Solid Edge part; units mm, degrees
sketch "Sketch1" plane through (0, 0, 0) normal (0, -1, 0) x (1, 0, 0)
  line L0 (-47.0022, 489.0599) -> (-22.0022, 514.0599)
  line L1 (-22.0022, 514.0599) -> (-22.0022, 81.0447)
  line L2 (-22.0022, 81.0447) -> (162.9162, 149.0358)
  line L3 (197.0498, 56.2011) -> (162.9162, 149.0358)
  line L4 (-113.6611, -58.0415) -> (197.0498, 56.2011)
  line L5 (-113.6611, -58.0415) -> (-140.1715, 14.0599)
  line L6 (-522.0022, 14.0599) -> (-140.1715, 14.0599)
  line L7 (-497.0022, 39.0599) -> (-522.0022, 14.0599)
  line L8 (-497.0022, 39.0599) -> (-147.0022, 39.0599)
  line L9 (-47.0022, 139.0599) -> (-147.0022, 39.0599)
  line L10 (-47.0022, 139.0599) -> (-47.0022, 489.0599)
  dimension "D1" = 497.0022
extrude "Protrusion1" add sketch "Sketch1" along normal blind 10
sketch "Sketch2" plane through (-272.0022, -10, 264.0599) normal (0, -1, 0) x (0, 0, 1)
  line L0 (-265.7843, 265.7843) -> (-209.2157, 209.2157)
  line L1 (-209.2157, 209.2157) -> (-202.1447, 216.2868)
  line L2 (-202.1447, 216.2868) -> (-258.7132, 272.8553)
  line L3 (-258.7132, 272.8553) -> (-265.7843, 265.7843)
  line L4 (209.2157, -209.2157) -> (265.7843, -265.7843)
  line L5 (265.7843, -265.7843) -> (272.8553, -258.7132)
  line L6 (272.8553, -258.7132) -> (216.2868, -202.1447)
  line L7 (216.2868, -202.1447) -> (209.2157, -209.2157)
  dimension "D1" = 265.7843
  dimension "D2" = 272.8553
  dimension "D3" = 209.2157
  dimension "D4" = 202.1447
extrude "ExtrudedProtrusion_2" add sketch "Sketch2" against normal blind 80
sketch "Sketch3" plane through (-173.9038, -10, 239.4369) normal (0, -1, 0) x (1, 0, 0)
  line L0 (289.8917, -107.6558) -> (324.0253, -200.4904)
  line L1 (324.0253, -200.4904) -> (370.9537, -183.2357)
  line L2 (370.9537, -183.2357) -> (336.8201, -90.401)
  line L3 (336.8201, -90.401) -> (289.8917, -107.6558)
  dimension "D1" = 336.8201
  dimension "D2" = 370.9537
extrude "ExtrudedProtrusion_3" add sketch "Sketch3" along normal blind 50
sketch "Sketch4" plane through (-66.322, 10, 476.8112) normal (-0.7071068, 0, -0.7071068) x (0, -1, 0)
  line L0 (20, 5) -> (39.0788, 11)
  line L1 (39.0788, 11) -> (39.0788, 1)
  line L2 (39.0788, 1) -> (20, -5)
  line L3 (20, -5) -> (20, 5)
  line L4 (-60, 5) -> (-79.0788, 11)
  line L5 (-79.0788, 11) -> (-79.0788, 1)
  line L6 (-79.0788, 1) -> (-60, -5)
  line L7 (-60, 5) -> (-60, -5)
  dimension "D1" = 79.0788
  dimension "D2" = 79.0788
  dimension "D3" = 79.0788
extrude "ExtrudedProtrusion_4" add sketch "Sketch4" against normal blind 80
sketch "Sketch5" plane through (-541.322, 30, 1.8112) normal (-0.7071068, 0, -0.7071068) x (0, -1, 0)
  line L0 (-40, 5) -> (-59.0788, 11)
  line L1 (-59.0788, 11) -> (-59.0788, 1)
  line L2 (-59.0788, 1) -> (-40, -5)
  line L3 (-40, -5) -> (-40, 5)
  line L4 (40, 5) -> (40, -5)
  line L5 (40, -5) -> (59.0788, 1)
  line L6 (59.0788, 1) -> (59.0788, 11)
  line L7 (59.0788, 11) -> (40, 5)
extrude "ExtrudedProtrusion_5" add sketch "Sketch5" against normal blind 80
sketch "Sketch6" plane through (133.0546, -35, 85.3638) normal (-0.9385681, 0, -0.3450941) x (0, -1, 0)
  line L0 (25, 49.4555) -> (25, -49.4555)
  line L1 (25, -49.4555) -> (7.5593, -49.4555)
  line L2 (7.5593, -49.4555) -> (25, 49.4555)
extrude "Cutout1" cut sketch "Sketch6" against normal through all
The listing builds one solid part. Answer for the finished solid, in the listing's coordinates (mm). A direction names the side the tool comes from. Give positions to 0.01 mm unless a question says otherwise; leave off trailing zeros. Order: outer loops, then holes, each group sorted by start corner. A loop starts at its lowest first (then second) coordinate and runs counter-clockwise, first axis right, second up. Notation, with made-up numbers: (72.5, 64.25) - (108.5, 64.25) arc R24 ccw to (108.5, 92.25) - close; hole circle Ø4 at (-18, -24). An arc over 180 degrees is marked (long way). Answer as CSV lines item,"result".
Q1. Each of these flat-tipped pins is pushed along its axis until it touches: pin 1 Ø8 at (y, z) = (-4, 354.5) entering from -X; pin 2 Ø5 at (y, z) = (-6, 228) entering from +X; pin 3 Ø5 at (x, y) = (-379.5, -6) entering from -Z. Where does it stop, or does it pass through?
Answer key:
pin 1,"stops at x = -47"
pin 2,"stops at x = -22"
pin 3,"stops at z = 14.06"
Q2. Which of the six approach directions +Z, -Z, +X, -X, +Y, -Y give full straight-line access (tool end or side, diameter ignored) to faces 5 (the face through (-519.06, 79.41, 35.33)), 6 (the face through (-43, 89.079, 509)), 7 (the face through (-511.99, -19.406, 28.255))?
Answer key:
face 5,"+Z, -X"
face 6,"+Z, -Z, +X, -X, +Y"
face 7,"-Z, -Y"
Q3. A cutting plane is placed at A-A, the plane y = 50.5. Determine the outline of the cut face in (x, z), and give its area (3 significant figures).
Answer key:
outline,"(-544.86, 5.35) - (-537.79, -1.72) - (-481.22, 54.84) - (-488.29, 61.92) - close; (-69.86, 480.35) - (-62.79, 473.28) - (-6.22, 529.84) - (-13.29, 536.92) - close"
area,"1,600 mm^2"
Q4. A cutting plane is placed at B-B, the plane x = -415.5. Determine the outline of the cut face in (y, z).
Answer key:
outline,"(-10, 14.06) - (0, 14.06) - (0, 39.06) - (-10, 39.06) - close"
Q5. Determine the mould class of faces 1 (the face through (-96.3, -4.93, 89.76)), 2 (the face through (-81, 0, 78)), 3 (the face through (-518, -29.079, 34)), 4 (the face through (-44.06, 79.41, 510.33)) for opening direction Y: pulls with the +Y half, pulls with the -Y half, needs draft (parallel to the pull), parting line crosses it, or undercut.
Answer key:
face 1,"needs draft"
face 2,"pulls with the +Y half"
face 3,"pulls with the -Y half"
face 4,"undercut"
Q6. A cutting plane is placed at C-C, the plane z = 180.5. Determine the outline of the cut face in (x, y).
Answer key:
outline,"(-47, -10) - (-22, -10) - (-22, 0) - (-47, 0) - close"
Q7. Straight lines are drawn through the part: L1, parallel to X at y = -8, z = 341.5; L2, parallel to Y at x = -27, z = 376. For each, find the intervals that lie inside material, in ascending order.
Answer key:
L1,"x = -47 to -22"
L2,"y = -10 to 0"
